Could you check a few things on this model? Use its own coordinates, in mm. A direction names the side the tool comes from. Coordinates: 2 decimals unless noted, no trailing zeros. Write each loop counter-clockwise with the first axis right and the second up, starting at its lowest first coordinate (ties: lowest second). Pieces come first, ordered by that corner, then holes. Notation, with made-up numbers: (30.5, -14.5) - (72.5, -14.5) arc R26 ccw to (72.5, 8.5) - close; hole circle Ø10 at (23.5, 65). An arc over 180 degrees is marked (long way). Write item = value, one per line. Start each with the question number.
```python
from build123d import *

# Parameters (mm, degrees)
SHELL1_OUTLINE_R = 15
SHELL1_DEPTH     = 30


# Read off the part's stored shape, not the designer's step: Shell1
with BuildPart() as part:
    # Sketch1 → Revolve1 (revolve)
    with BuildSketch(Plane.XY):
        Polygon((0, 35), (35, 35), (35, 25), (20, 25), (20, 0), (0, 0), align=None)
    revolve(axis=Axis((0, 0, 0), (0, 1, 0)))

    # Shell1 outline → Shell1 (cut)
    with BuildSketch(Plane(origin=(0, 0, 0), x_dir=(1, 0, 0), z_dir=(0, 1, 0))):
        Circle(SHELL1_OUTLINE_R)
    extrude(amount=SHELL1_DEPTH, mode=Mode.SUBTRACT)


solid = part.part
```
1) Which directions (+Z, -Z, +X, -X, +Y, -Y) give clear straight access to the entire face, cutting with the end or side of a thin tool? Please do faces 5 (the flat face through (15, 25, 15)), 6 (the flat face through (0, 35, 0)).
2) Suppose I cut it at A-A on z = 0. Please give me the cut outline in (x, y).
3) For P1, Ø4, axis at y = 15, z = 12, coming from the +X side; P2, Ø5, axis at y = 11, z = 20.5, coming from the -X side; P3, Ø8, axis at x = 1, y = 13.5, coming from the +Z side, each with a flat end and sliding along its axis, tell me the tip position at first contact or that it passes through.
4) Suppose I cut it at D-D on y = 8. Please give me the cut outline in (x, z), plus the area to 3 significant figures.
5) Suppose I cut it at C-C on y = 27. Please give me the cut outline in (x, z), plus the area to 3 significant figures.
6) Suppose I cut it at B-B on x = 0. Please give me the cut outline in (y, z).
7) Thinking about a two-plate mould opening in X: for faces 1 (the flat face through (3, 0, -15)), 2 (the flat face through (0, 30, 0)), 3 (the cylindrical face through (-14.985, 14.79, -0.66)), 4 (the cylindrical face through (-28, 30, 21)), which applies, +X half, -X half, draft (parallel to the pull), parting line (faces both ways), or undercut?
8) If I drill on probe 1 along X at (y, z) = (24, 0); probe 2 along Y at (x, z) = (5, -25), over which ranges is the centre line in solid material (lowest first)? Write a range as [from, to].
Reply:
q1.face_5 = -Y
q1.face_6 = +Z, -Z, +X, -X, +Y
q2.outline = (-35, 25) - (-20, 25) - (-20, 0) - (-15, 0) - (-15, 30) - (15, 30) - (15, 0) - (20, 0) - (20, 25) - (35, 25) - (35, 35) - (-35, 35) - close
q3.P1 = 17.32
q3.P2 = -8.72
q3.P3 = 20
q4.outline = circle Ø40 at (0, 0); hole circle Ø30 at (0, 0)
q4.area = 550 mm^2
q5.outline = circle Ø70 at (0, 0); hole circle Ø30 at (0, 0)
q5.area = 3,140 mm^2
q6.outline = (0, -20) - (25, -20) - (25, -35) - (35, -35) - (35, 35) - (25, 35) - (25, 20) - (0, 20) - (0, 15) - (30, 15) - (30, -15) - (0, -15) - close
q7.face_1 = draft
q7.face_2 = undercut
q7.face_3 = undercut
q7.face_4 = parting line
q8.probe_1 = [-20, -15], [15, 20]
q8.probe_2 = [25, 35]
